For this review, take the finished solid that the model builds, in its own axes (mm). A direction names the side the tool comes from. Round coordinates to 2 decimals unless told otherwise and drop trailing zeros. Loops run counter-clockwise (first coordinate to the right, second up) from the corner with the lowest first, then second, coordinate; pieces in that order, holes last. Notation, with made-up numbers: M 32,50 L 82,50 A21 cw 82,66 Z; hole C 37.25,36 d11. An arc over 180 degrees is marked long. One line per question, with ' | ' between items. Start each with the question number.
1) We need section C-C (z = -6.5). Give the boundary of the cut face in (x, y).
2) Mouldability with a two-part tool opening along Y and no side actions: class faces 6 (the face through (65, 65, -20)), 7 (the face through (65, 65, 20)), 8 (the face through (45, 32, 0)), 9 (the face through (42, 55, 25)) as pulls with the +Y half, pulls with the -Y half, needs draft (parallel to the pull), parting line crosses it, or undercut.
3) For faces 1 (the face through (-5, 20, -9)), 2 (the face through (35, 40, 23)), 3 (the face through (40, 34, -15)), 4 (the face through (58, 35, 0)), 5 (the face through (24, 10, 0)), list the 3-axis set-ups (+Z, -Z, +X, -X, +Y, -Y) from which the entire face can be reached by the end or side of a thin tool; tool diameter is ignored.
4) We need section D-D (x = 65). Give the boundary of the cut face in (y, z).
5) For probe 1 along X at (y, z) = (22.1, 0); probe 2 along Z at (x, y) = (0, 12); probe 3 along X at (y, z) = (97.5, 0), list the stretches that pass through material, from the lowest coordinate up. Write a range as from..to.
6) For pin 1 Ø8 at (x, z) = (43.5, 26) entering from +Y; pin 2 Ø1.5 at (y, z) = (14.5, -4.5) entering from -X; pin 3 Ø5 at (x, z) = (33.5, -3) entering from +Y, all flat-tipped, find the tip position at first contact; note any pin that passes through.
7) We need section B-B (y = 81). Give the boundary of the cut face in (x, z), and give its area (3 significant figures).
8) We need section A-A (z = 0). Give the boundary of the cut face in (x, y), and give its area (3 significant figures).
```python
from build123d import *

# Parameters (mm, degrees)
SKETCH1_R               = 10
BOSS_EXTRUDE1_DEPTH     = 25
BOSS_EXTRUDE2_DEPTH     = 45
SKETCH4_W               = 110
SKETCH4_H               = 10
CUT_EXTRUDE1_DEPTH      = 12.5
SKETCH5_W               = 15
SKETCH5_H               = 50
CUT_EXTRUDE2_DEPTH      = 32.5
SKETCH6_W               = 10
SKETCH6_H               = 30
CUT_EXTRUDE3_DEPTH      = 65
CUT_EXTRUDE3_DEPTH_BACK = 30
SKETCH7_R               = 20
CUT_EXTRUDE4_DEPTH      = 5
SKETCH9_R               = 2.5
CUT_EXTRUDE5_DEPTH      = 55


with BuildPart() as part:
    # Sketch1 → Boss-Extrude1 (new body)
    with BuildSketch(Plane(origin=(0, 0, 0), x_dir=(1, 0, 0), z_dir=(0, 1, 0))):
        with BuildLine():
            Line((0, -30), (80, -30))
            Line((80, -30), (80, 30))
            Line((80, 30), (0, 30))
            ThreePointArc((0, 30), (-30, 0), (0, -30))
        make_face()
        Circle(SKETCH1_R, mode=Mode.SUBTRACT)
    extrude(amount=BOSS_EXTRUDE1_DEPTH)

    # Sketch2 → Boss-Extrude2 (add)
    with BuildSketch(Plane(origin=(80, 0, 0), x_dir=(0, 0, -1), z_dir=(1, 0, 0))):
        with BuildLine():
            Line((-30, 25), (30, 25))
            Line((30, 25), (30, 75))
            Line((30, 75), (20, 75))
            Line((20, 75), (20, 55))
            ThreePointArc((20, 55), (0, 35), (-20, 55))
            Line((-20, 55), (-20, 75))
            Line((-20, 75), (-30, 75))
            Line((-30, 75), (-30, 25))
        make_face()
        with BuildLine():
            Line((20, 75), (30, 75))
            ThreePointArc((30, 75), (0, 105), (-30, 75))
            Line((-30, 75), (-20, 75))
            ThreePointArc((-20, 75), (-17.020295968, 85.502834149), (-8.969047485, 92.876134572))
            ThreePointArc((-8.969047485, 92.876134572), (2.405486487, 94.854813894), (12.978420983, 90.217114995))
            ThreePointArc((12.978420983, 90.217114995), (18.159961724, 83.379486271), (20, 75))
        make_face()
    extrude(amount=-BOSS_EXTRUDE2_DEPTH)

    # Sketch4 → Cut-Extrude1 (cut, symmetric)
    with BuildSketch(Plane.XY):
        with Locations((25, 5)):
            Rectangle(SKETCH4_W, SKETCH4_H)
    extrude(amount=CUT_EXTRUDE1_DEPTH, both=True, mode=Mode.SUBTRACT)

    # Sketch5 → Cut-Extrude2 (cut, symmetric)
    with BuildSketch(Plane.XY):
        with Locations((42.5, 80)):
            Rectangle(SKETCH5_W, SKETCH5_H)
    extrude(amount=CUT_EXTRUDE2_DEPTH, both=True, mode=Mode.SUBTRACT)

    # Sketch6 → Cut-Extrude3 (cut, two sides)
    with BuildSketch(Plane(origin=(0, 55, 0), x_dir=(1, 0, 0), z_dir=(0, 1, 0))) as cut_extrude3_sk:
        with Locations((40, 0)):
            Rectangle(SKETCH6_W, SKETCH6_H)
    extrude(amount=CUT_EXTRUDE3_DEPTH, mode=Mode.SUBTRACT)
    extrude(cut_extrude3_sk.sketch, amount=-CUT_EXTRUDE3_DEPTH_BACK, mode=Mode.SUBTRACT)

    # Sketch7 → Cut-Extrude4 (cut)
    with BuildSketch(Plane(origin=(0, 25, 0), x_dir=(1, 0, 0), z_dir=(0, 1, 0))):
        Circle(SKETCH7_R)
    extrude(amount=-CUT_EXTRUDE4_DEPTH, mode=Mode.SUBTRACT)

    # Sketch9 → Cut-Extrude5 (cut)
    with BuildSketch(Plane(origin=(0, 55, 0), x_dir=(1, 0, 0), z_dir=(0, 1, 0))):
        with Locations((65, 0)):
            Circle(SKETCH9_R)
    extrude(amount=CUT_EXTRUDE5_DEPTH, mode=Mode.SUBTRACT)


solid = part.part
```
Answers below:
1) outline: M -29.29,10 L -7.6,10 L -7.6,20 L -18.91,20 L -18.91,25 L -29.29,25 Z; M 7.6,10 L 80,10 L 80,36.09 L 45,36.09 L 45,25 L 18.91,25 L 18.91,20 L 7.6,20 Z; M 50,93.91 L 80,93.91 L 80,104.29 L 50,104.29 Z
2) face 6: undercut | face 7: undercut | face 8: needs draft | face 9: pulls with the +Y half
3) face 1: +Y | face 2: +Z, -Z, -X, +Y | face 3: -X, +Y | face 4: +X, -X | face 5: +X, -X, -Y
4) outline: M 0,-30 L 75,-30 A30 ccw 104.9,-2.5 L 94.84,-2.5 A20 cw 75,-20 L 55,-20 A20 cw 55,20 L 75,20 A20 cw 94.84,2.5 L 104.9,2.5 A30 ccw 75,30 L 0,30 L 0,12.5 L 10,12.5 L 10,-12.5 L 0,-12.5 Z
5) probe 1: -30..-20, 20..80 | probe 2: -30..-10, 10..30 | probe 3: 50..62.5, 67.5..80
6) pin 1: y = 55 | pin 2: x = -29.76 | pin 3: y = 25
7) outline: M 50,-29.39 L 80,-29.39 L 80,-19.08 L 50,-19.08 Z; M 50,19.08 L 80,19.08 L 80,29.39 L 50,29.39 Z | area: 619 mm^2
8) outline: M -30,10 L -10,10 L -10,20 L -20,20 L -20,25 L -30,25 Z; M 10,10 L 80,10 L 80,35 L 45,35 L 45,25 L 20,25 L 20,20 L 10,20 Z; M 50,95 L 62.5,95 L 62.5,105 L 50,105 Z; M 67.5,95 L 80,95 L 80,105 L 67.5,105 Z | area: 1,850 mm^2
